from build123d import *

# Parameters (mm, degrees)
PAD032_DEPTH    = 19.05
SKETCH066_R     = 2.286
POCKET002_DEPTH = 6.223
SKETCH067_R     = 2.286
POCKET003_DEPTH = 6.223
SKETCH068_R     = 1.651
PAD041_DEPTH    = 3.175


with BuildPart() as part:
    # Sketch065 → Pad032 (new body)
    with BuildSketch(Plane.YZ):
        with BuildLine():
            Line((-19.05, 9.525), (-19.05, -9.525))
            Line((-19.05, -9.525), (19.05, -9.525))
            Line((19.05, -9.525), (19.05, 9.525))
            Line((19.05, 9.525), (12.375, 9.525))
            ThreePointArc((-12.375, 9.525), (0, -2.85), (12.375, 9.525))
            Line((-12.375, 9.525), (-19.05, 9.525))
        make_face()
    extrude(amount=PAD032_DEPTH)

    # Sketch066 (on Face6 of Pad032) → Pocket002 (cut)
    with BuildSketch(Plane(origin=(0, 0, 9.525), x_dir=(0, -1, 0), z_dir=(0, 0, 1))):
        with Locations((15.875, 15.875)):
            Circle(SKETCH066_R)
        with Locations((15.875, 3.175)):
            Circle(SKETCH066_R)
        with Locations((-15.875, 15.875)):
            Circle(SKETCH066_R)
        with Locations((-15.875, 3.175)):
            Circle(SKETCH066_R)
    extrude(amount=-POCKET002_DEPTH, mode=Mode.SUBTRACT)

    # Sketch067 (on Face2 of Pad032) → Pocket003 (cut)
    with BuildSketch(Plane.YX.offset(9.525)):
        with Locations((15.875, 15.875)):
            Circle(SKETCH067_R)
        with Locations((15.875, 3.175)):
            Circle(SKETCH067_R)
        with Locations((-15.875, 15.875)):
            Circle(SKETCH067_R)
        with Locations((-15.875, 3.175)):
            Circle(SKETCH067_R)
    extrude(amount=-POCKET003_DEPTH, mode=Mode.SUBTRACT)

    # Sketch068 (on Face5 of Pocket003) → Pad041 (join)
    with BuildSketch(Plane.YZ.offset(19.05)):
        with BuildLine():
            Line((-19.05, -9.525), (19.05, -9.525))
            Line((19.05, -9.525), (19.05, 22.225))
            Line((19.05, 22.225), (9.525, 22.225))
            Line((9.525, 22.225), (4.445, 9.525))
            ThreePointArc((-4.445, 9.525), (0, 5.08), (4.445, 9.525))
            Line((-9.525, 22.225), (-4.445, 9.525))
            Line((-19.05, 22.225), (-9.525, 22.225))
            Line((-19.05, -9.525), (-19.05, 22.225))
        make_face()
        with Locations((-8.509, 9.525)):
            Circle(SKETCH068_R, mode=Mode.SUBTRACT)
        with Locations((8.509, 9.525)):
            Circle(SKETCH068_R, mode=Mode.SUBTRACT)
    extrude(amount=PAD041_DEPTH)


with BuildPart() as part_1:
    # Body026 placement: moved
    add(part.part.moved(Location((-21.5138, 40.6146, -8.9154))))


solid = part_1.part
Design review of the part built by this model. Coordinates are the model's own, in mm. A direction names the side the tool comes from. Coordinates: 2 decimals unless noted, no trailing zeros. Order: outer loops, then holes, each group sorted by start corner. A loop starts at its lowest first (then second) coordinate and runs counter-clockwise, first axis right, second up. Notation, with made-up numbers: (61, 3.25) - (89, 3.25) arc R26 ccw to (89, 36.25) - close; hole circle Ø9 at (-32.75, -3.75). An arc over 180 degrees is marked (long way). Put each result on its own line as item: value.
1) Insertion check: P1, Ø1.4, axis at x = -5.5, y = 56, coming from the +Z side; P2, Ø2.5, axis at x = -17.5, y = 24.5, coming from the -Z side; P3, Ø7.5, axis at x = -12, y = 56.5, coming from the +Z side. Each pin has a flat end and moves straight along its axis. Give the tip position at first contact, or say it passes through.
Response values:
P1: stops at z = -5.61
P2: stops at z = -12.22
P3: stops at z = 0.61
2) Take a section at D-D, the plane z = -5. Give the boundary of the cut face in (x, y).
Response values:
outline: (-21.51, 21.56) - (0.71, 21.56) - (0.71, 59.66) - (-21.51, 59.66) - (-21.51, 51.65) - (-2.46, 51.65) - (-2.46, 29.58) - (-21.51, 29.58) - close; hole circle Ø4.57 at (-18.34, 24.74); hole circle Ø4.57 at (-18.34, 56.49); hole circle Ø4.57 at (-5.64, 24.74); hole circle Ø4.57 at (-5.64, 56.49)
3) Tool access review of faces 4 (the face through (-12, 25, 0.61)), 5 (the face through (-18, 25, -12.217)), 6 (the face through (-6, 57, -5.613)), 7 (the face through (-0.899, 33.594, 7.049)), 8 (the face through (-11, 40, -18.44)): name each direction out of +Z, -Z, +X, -X, +Y, -Y from which nothing blocks a thin tool from reaching the whole face with its end or side.
Response values:
face 4: +Z, -X, +Y, -Y
face 5: -Z
face 6: +Z
face 7: +Z, +X, -X
face 8: -Z, +X, -X, +Y, -Y
4) The part is to be moulded in two halves that separate along X. For faces 1 (the face through (-12.122, 40.342, -11.762)), 2 (the face through (-18, 57, -5.613)), 3 (the face through (-21.514, 40, -13)), say which applies: released by +X, released by -X, zero draft, split by the parting line, or undercut.
Response values:
face 1: zero draft
face 2: undercut
face 3: released by -X
5) Wall thickness on L1, parallel to X at y = 56.5, z = -4.5; L2, parallel to Y at x = -17.75, z = -3; L3, parallel to X at y = 26, z = -5: over which ranges is each line inside the solid? List them lowest first. Write a range as from..to.
Response values:
L1: x = -21.51..-20.62, -16.05..-7.92, -3.35..0.71
L2: y = 21.56..22.53, 26.95..28.78, 52.45..54.28, 58.7..59.66
L3: x = -21.51..-20.25, -16.43..-7.55, -3.73..0.71
6) Take a section at C-C, the plane x = -12.5. Give the boundary of the cut face in (y, z) (3 decimals).
Response values:
outline: (21.565, -18.44) - (59.665, -18.44) - (59.665, 0.61) - (52.99, 0.61) arc R12.375 cw to (28.24, 0.61) - (21.565, 0.61) - close
7) Take a section at A-A, the plane z = 7.5. Give the boundary of the cut face in (x, y), and give its area (3 significant figures).
Response values:
outline: (-2.46, 21.56) - (0.71, 21.56) - (0.71, 33.41) - (-2.46, 33.41) - close; (-2.46, 47.82) - (0.71, 47.82) - (0.71, 59.66) - (-2.46, 59.66) - close
area: 75.2 mm²
8) Take a section at B-B, the plane y = 32.5. Give the boundary of the cut face in (x, z).
Response values:
outline: (-21.51, -18.44) - (0.71, -18.44) - (0.71, -0.99) - (-2.46, -0.99) - (-2.46, -8.73) - (-21.51, -8.73) - close; (-2.46, 2.21) - (0.71, 2.21) - (0.71, 9.78) - (-2.46, 9.78) - close
